For this review, take the finished solid that the model builds, in its own axes (mm). Round coordinates to 2 decimals unless told otherwise and drop trailing zeros. Write each loop counter-clockwise with the first axis right and the second up, starting at its lowest first coordinate (ties: lowest second). Pieces come first, ordered by that corner, then holes. Notation, with made-up numbers: (-19, 51.5) -> (30, 51.5) arc R9 ccw to (30, 58.5) -> close; hole circle Ø8 at (13, -33). An arc over 180 degrees is marked (long way). Answer in a Markdown table with one row per item.
from build123d import *

# Parameters (mm, degrees)
F1_DEPTH = 7
F2_R     = 7.5
F3_DEPTH = 47.6


with BuildPart() as f1:
    # F0 (on Front) → F1 (new body)
    with BuildSketch(Plane.XZ):
        with BuildLine():
            ThreePointArc((0, 11.125), (7.866563, 7.866563), (11.125, 0))
            ThreePointArc((11.125, 0), (10.745925, -2.879362), (9.634533, -5.5625))
            Line((9.634533, -5.5625), (30.419142, -17.5625))
            ThreePointArc((30.419142, -17.5625), (31.137901, -7.928761), (24.049755, -1.364942))
            ThreePointArc((24.049755, -1.364942), (11.696795, 6.753148), (10.842803, 21.51017))
            ThreePointArc((10.842803, 21.51017), (8.702442, 30.930594), (0, 35.125))
            Line((0, 35.125), (0, 11.125))
        make_face()
        with BuildLine():
            ThreePointArc((-9.634533, -5.5625), (-9.634533, 5.5625), (0, 11.125))
            Line((0, 11.125), (0, 35.125))
            ThreePointArc((0, 35.125), (-8.702442, 30.930594), (-10.842803, 21.51017))
            ThreePointArc((-10.842803, 21.51017), (-10.660456, 20.918313), (-10.498883, 20.32045))
            ThreePointArc((-10.498883, 20.32045), (-12.339117, 7.123992), (-22.847468, -1.067926))
            ThreePointArc((-22.847468, -1.067926), (-23.446018, -1.226931), (-24.049755, -1.364942))
            ThreePointArc((-24.049755, -1.364942), (-31.137901, -7.928761), (-30.419142, -17.5625))
            Line((-30.419142, -17.5625), (-9.634533, -5.5625))
        make_face()
        with BuildLine():
            Line((30.419142, -17.5625), (9.634533, -5.5625))
            ThreePointArc((9.634533, -5.5625), (0, -11.125), (-9.634533, -5.5625))
            Line((-9.634533, -5.5625), (-30.419142, -17.5625))
            ThreePointArc((-30.419142, -17.5625), (-22.435459, -23.001833), (-13.206952, -20.145228))
            ThreePointArc((-13.206952, -20.145228), (0, -15.150958), (13.206952, -20.145228))
            ThreePointArc((13.206952, -20.145228), (22.435459, -23.001833), (30.419142, -17.5625))
        make_face()
        with BuildLine():
            ThreePointArc((-10.498883, 20.32045), (-10.660456, 20.918313), (-10.842803, 21.51017))
            ThreePointArc((-10.842803, 21.51017), (-10.68741, 20.910521), (-10.498883, 20.32045))
        make_face()
        with BuildLine():
            ThreePointArc((-22.847468, -1.067926), (-23.452747, -1.199691), (-24.049755, -1.364942))
            ThreePointArc((-24.049755, -1.364942), (-23.446018, -1.226931), (-22.847468, -1.067926))
        make_face()
    extrude(amount=F1_DEPTH)

    # F2 (on Front) → F3 (cut)
    with BuildSketch(Plane.XZ):
        with Locations((20.449737, -11.921206)):
            Circle(F2_R)
        with Locations((-21.451427, -12.500484)):
            Circle(F2_R)
        with Locations((0, 25.152633)):
            Circle(F2_R)
    extrude(amount=F3_DEPTH, mode=Mode.SUBTRACT)


solid = f1.part
1) Consider section C-C on y = -4.5. State how many separate pieces and enclosed holes the cut face has, then the cut area to 3 significant figures.
Solved:
| item | result |
|---|---|
| separate pieces | 1 |
| enclosed holes | 4 |
| area | 1,010 mm² |
2) For line 1 (Z direction, x = -5, y = -0.25); line 2 (X direction, y = -4, z = -8); line 3 (Z direction, x = -4, y = -1.25), list the stretches that pass through material, from the lowest coordinate up. Write a range as [from, to].
Solved:
| item | result |
|---|---|
| line 1 | [-15.79, -9.94], [9.94, 19.56], [30.74, 33.94] |
| line 2 | [-31.17, -27.45], [-15.45, -7.73], [7.73, 14.06], [26.84, 31.17] |
| line 3 | [-15.56, -10.38], [10.38, 18.81], [31.5, 34.38] |
3) Mouldability with a two-part tool opening along X and no side actions: class faces 1 (the cylindrical face through (-1.63, -3.45, 17.83)), 2 (the flat face through (-3, -7, -11)), 3 (the cylindrical face through (-12.244, -3.451, 7.29)), 4 (the cylindrical face through (11.805, -3.451, 6.568)) as pulls with the +X half, pulls with the -X half, needs draft (parallel to the pull), parting line crosses it, or undercut.
Solved:
| item | result |
|---|---|
| face 1 | undercut |
| face 2 | needs draft |
| face 3 | pulls with the -X half |
| face 4 | pulls with the +X half |
4) Consider section B-B on x = 19. State the section outline as (y, z) points, then the cut area to 3 significant figures.
Solved:
| item | result |
|---|---|
| outline | (-7, -22.98) -> (0, -22.98) -> (0, -19.28) -> (-7, -19.28) -> close; (-7, -4.56) -> (0, -4.56) -> (0, 0.06) -> (-7, 0.06) -> close |
| area | 58.3 mm² |
5) Consider section A-A on z = 26.5. State the section outline as (x, y) points, then the cut area to 3 significant figures.
Solved:
| item | result |
|---|---|
| outline | (-10.84, -7) -> (-7.38, -7) -> (-7.38, 0) -> (-10.84, 0) -> close; (7.38, -7) -> (10.84, -7) -> (10.84, 0) -> (7.38, 0) -> close |
| area | 48.5 mm² |
6) Clearance check with flat-ended pins moving along their axes: pin 1 Ø12 at (x, z) = (0, 25.15) entering from +Y; pin 2 Ø4 at (y, z) = (-1.5, 13) entering from -X; pin 3 Ø2 at (y, z) = (-4, -1.5) entering from -X; pin 4 Ø2 at (y, z) = (-5, -7) entering from -X. State where each tip first meets the part, or that it passes through.
Solved:
| item | result |
|---|---|
| pin 1 | through |
| pin 2 | x = -10.68 |
| pin 3 | x = -26.57 |
| pin 4 | x = -31.17 |
